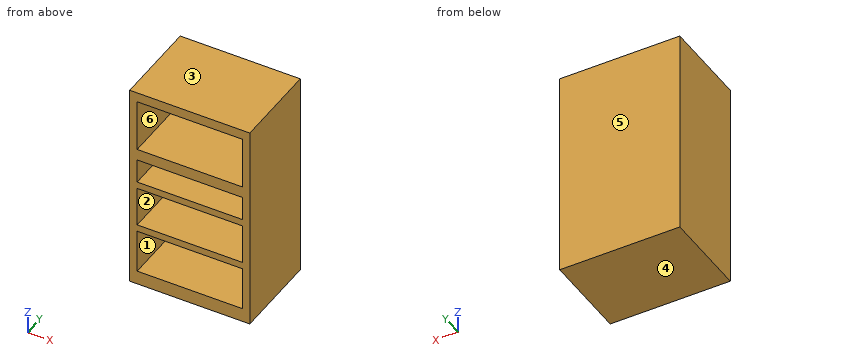
from build123d import *

# Parameters (mm, degrees)
F0_W     = 87.015488
F0_H     = 152.645812
F1_DEPTH = 12.7
F2_W     = 87.015488
F2_H     = 152.645812
F2_W_2   = 76.2
F2_H_2   = 38.1
F3_DEPTH = 50.8
F2_H_3   = 5.08
F4_DEPTH = 50.8


with BuildPart() as f1:
    # F0 (on Front) → F1 (new body)
    with BuildSketch(Plane.XZ):
        Rectangle(F0_W, F0_H)
    extrude(amount=F1_DEPTH)

    # F2 (on face) → F3 (join)
    with BuildSketch(Plane.XZ.offset(12.7)):
        Rectangle(F2_W, F2_H)
        Polygon((-38.1, 22.737094), (38.1, 22.737094), (38.1, 5.08), (38.1, 0), (38.1, -29.176182), (38.1, -34.256182), (38.1, -66.162906), (-38.1, -66.162906), (-38.1, -34.256182), (-38.1, -29.176182), (-38.1, 0), (-38.1, 5.08), align=None, mode=Mode.SUBTRACT)
        with Locations((0, 50.189414)):
            Rectangle(F2_W_2, F2_H_2, mode=Mode.SUBTRACT)
    extrude(amount=F3_DEPTH)

    # F2 (on face) → F4 (join)
    with BuildSketch(Plane.XZ.offset(12.7)):
        with Locations((0, 2.54)):
            Rectangle(F2_W_2, F2_H_3)
        with Locations((0, -31.716182)):
            Rectangle(F2_W_2, F2_H_3)
    extrude(amount=F4_DEPTH)


solid = f1.part
Geometry check sheet. Reference: the model listing, model coordinates, mm. Face numbers are marked on the shaded views. A direction names the side the tool comes from. Coordinates: 2 decimals unless noted, no trailing zeros. Order: outer loops, then holes, each group sorted by start corner. A loop starts at its lowest first (then second) coordinate and runs counter-clockwise, first axis right, second up. Notation, with made-up numbers: (69.5, 72) - (89.5, 72) arc R12 cw to (89.5, 85) - close; hole circle Ø10 at (18, 9). An arc over 180 degrees is marked (long way). Answer in a Markdown table with one row per item. Add a question column.
1) Cross-section at B-B, the plane z = -60. Record the cut outline in (x, y), then the cut area to 3 significant figures.
2) Gauge pin test, flat end, axial feed: P1, Ø5.5, axis at x = 18, z = 12.5, coming from the -Y side. Record the tip position at first contact, or that the pin passes through.
3) Cross-section at C-C, the plane x = -4. Record the cut outline in (y, z).
4) Cross-section at A-A, the plane y = -48. Record the cut outline in (x, z), then the cut area to 3 significant figures.
5) Material ranges on line 1 along Z through (x, y) = (-3.5, -58); line 2 along X through (y, z) = (-41.5, 68.5); line 3 along Y through (x, z) = (-6, 42), recorded low to high. Write a range as [from, to].
6) Set-up check for the marked faces 5 and 6: record each of +Z, -Z, +X, -X, +Y, -Y from which the full face is reachable in a straight line by a thin tool's end or side.
7) Release check for a two-part mould opening along Z. For the marked faces 1, 2, 3 and 4 record: +Z half, -Z half, draft (parallel to the pull), parting line (faces both ways), or undercut.
Check result:
| question | item | result |
|---|---|---|
| 1 | outline | (-43.51, -63.5) - (-38.1, -63.5) - (-38.1, -12.7) - (38.1, -12.7) - (38.1, -63.5) - (43.51, -63.5) - (43.51, 0) - (-43.51, 0) - close |
| 1 | area | 1,650 mm² |
| 2 | P1 | stops at y = -12.7 |
| 3 | outline | (-63.5, -76.32) - (0, -76.32) - (0, 76.32) - (-63.5, 76.32) - (-63.5, 69.24) - (-12.7, 69.24) - (-12.7, 31.14) - (-63.5, 31.14) - (-63.5, 22.74) - (-12.7, 22.74) - (-12.7, 5.08) - (-63.5, 5.08) - (-63.5, 0) - (-12.7, 0) - (-12.7, -29.18) - (-63.5, -29.18) - (-63.5, -34.26) - (-12.7, -34.26) - (-12.7, -66.16) - (-63.5, -66.16) - close |
| 4 | outline | (-43.51, -76.32) - (43.51, -76.32) - (43.51, 76.32) - (-43.51, 76.32) - close; hole (-38.1, -66.16) - (38.1, -66.16) - (38.1, -34.26) - (-38.1, -34.26) - close; hole (-38.1, -29.18) - (38.1, -29.18) - (38.1, 0) - (-38.1, 0) - close; hole (-38.1, 5.08) - (38.1, 5.08) - (38.1, 22.74) - (-38.1, 22.74) - close; hole (-38.1, 31.14) - (38.1, 31.14) - (38.1, 69.24) - (-38.1, 69.24) - close |
| 4 | area | 4,380 mm² |
| 5 | line 1 | z = [-76.32, -66.16], [-34.26, -29.18], [0, 5.08], [22.74, 31.14], [69.24, 76.32] |
| 5 | line 2 | x = [-43.51, -38.1], [38.1, 43.51] |
| 5 | line 3 | y = [-12.7, 0] |
| 6 | face 5 | +Z, -Z, +X, -X, +Y |
| 6 | face 6 | -Y |
| 7 | face 1 | undercut |
| 7 | face 2 | undercut |
| 7 | face 3 | +Z half |
| 7 | face 4 | -Z half |
